Geometry: final body of the model. Coordinates: model frame, mm. A direction names the side the tool comes from. Coordinates: 2 decimals unless noted, no trailing zeros. Order: outer loops, then holes, each group sorted by start corner. A loop starts at its lowest first (then second) coordinate and runs counter-clockwise, first axis right, second up. Notation, with made-up numbers: M -40,67 L -9,67 A21 cw -9,81 Z; hole C 5.25,56.25 d7. An arc over 180 degrees is marked long. Write item = value, one per line.
from build123d import *

# Parameters (mm, degrees)
SKETCH1_R           = 17.35
BOSS_EXTRUDE1_DEPTH = 2.5
SKETCH2_R           = 4.35
CUT_EXTRUDE1_DEPTH  = 25.663637201
SKETCH3_R           = 1.25
CUT_EXTRUDE2_DEPTH  = 25.663637201
CUT_EXTRUDE3_DEPTH  = 25.663637201


with BuildPart() as part:
    # Sketch1 → Boss-Extrude1 (new body)
    with BuildSketch(Plane(origin=(0, 0, 0), x_dir=(1, 0, 0), z_dir=(0, 1, 0))):
        with Locations(Location((0, 0, 0), (0, 0, 270))):
            Circle(SKETCH1_R)
    extrude(amount=BOSS_EXTRUDE1_DEPTH)

    # Sketch2 → Cut-Extrude1 (cut, through all)
    with BuildSketch(Plane(origin=(0, 2.5, 0), x_dir=(1, 0, 0), z_dir=(0, 1, 0))):
        with Locations(Location((0, 0, 0), (0, 0, 270))):
            Circle(SKETCH2_R)
    extrude(amount=-CUT_EXTRUDE1_DEPTH, mode=Mode.SUBTRACT)

    # Sketch3 → Cut-Extrude2 (cut, through all)
    with BuildSketch(Plane(origin=(0, 2.5, 0), x_dir=(1, 0, 0), z_dir=(0, 1, 0))):
        with Locations(Location((-14.5, 0, 0), (0, 0, 270))):
            Circle(SKETCH3_R)
        with Locations(Location((14.5, 0, 0), (0, 0, 270))):
            Circle(SKETCH3_R)
    extrude(amount=-CUT_EXTRUDE2_DEPTH, mode=Mode.SUBTRACT)

    # Sketch4 → Cut-Extrude3 (cut, through all)
    with BuildSketch(Plane(origin=(0, 2.5, 0), x_dir=(1, 0, 0), z_dir=(0, 1, 0))):
        with BuildLine():
            Line((-4, -1.7095321), (-10, -14.17824037))
            ThreePointArc((-10, -14.17824037), (0, -17.35), (10, -14.17824037))
            Line((10, -14.17824037), (4, -1.7095321))
            ThreePointArc((4, -1.7095321), (0, -4.35), (-4, -1.7095321))
        make_face()
    extrude(amount=-CUT_EXTRUDE3_DEPTH, mode=Mode.SUBTRACT)


solid = part.part
1) Line query: L1, parallel to X at y = 1.95, z = 0; L2, parallel to X at y = 0.6, z = -0.5; L3, parallel to X at y = 0.7, z = 11. Output: solid intervals per line, ascending.
Numbers:
L1 = -17.35 to -15.75, -13.25 to -4.35, 4.35 to 13.25, 15.75 to 17.35
L2 = -17.34 to -15.65, -13.35 to -4.32, 4.32 to 13.35, 15.65 to 17.34
L3 = -13.42 to -8.47, 8.47 to 13.42
2) Set-up query: faces 1 (the face through (7.04, 1.27, 8.03)), 2 (the face through (15.74, 1.27, -0.16)). Return all of +Z, -Z, +X, -X, +Y, -Y with unobstructed straight access to the full face (end or side cutting, diameter ignored); none if empty.
Numbers:
face_1 = +Z, +Y, -Y
face_2 = +Y, -Y
3) Section B-B, the plane x = 14.5. Return loops of the section in (y, z), and give its area (3 significant figures).
Numbers:
outline = M 0,-9.53 L 2.5,-9.53 L 2.5,-1.25 L 0,-1.25 Z; M 0,1.25 L 2.5,1.25 L 2.5,9.53 L 0,9.53 Z
area = 41.4 mm²
4) Section A-A, the plane z = 0. Return loops of the section in (x, y), and give its area (3 significant figures).
Numbers:
outline = M -17.35,0 L -15.75,0 L -15.75,2.5 L -17.35,2.5 Z; M -13.25,0 L -4.35,0 L -4.35,2.5 L -13.25,2.5 Z; M 4.35,0 L 13.25,0 L 13.25,2.5 L 4.35,2.5 Z; M 15.75,0 L 17.35,0 L 17.35,2.5 L 15.75,2.5 Z
area = 52.5 mm²
5) Mould query, pull axis X, two halves, no side actions, for faces 3 (the face through (-13.26, 1.27, -0.16)), 4 (the face through (0.61, 1.23, -17.34)), 5 (the face through (-6.96, 1.27, 7.86)), 6 (the face through (0, 2.5, -5)). Classes: pulls with the +X half, pulls with the -X half, needs draft (parallel to the pull), parting line crosses it, or undercut.
Numbers:
face_3 = undercut
face_4 = parting line crosses it
face_5 = undercut
face_6 = needs draft
6) Section C-C, the plane z = 8. Return loops of the section in (x, y).
Numbers:
outline = M -15.4,0 L -7.03,0 L -7.03,2.5 L -15.4,2.5 Z; M 7.03,0 L 15.4,0 L 15.4,2.5 L 7.03,2.5 Z
7) Pin query (flat end, axial travel): pin 1 (5 mm diameter, centred on x = 0, z = 0, fed in from -Y); pin 2 (1 mm diameter, centred on y = 1, z = -3.5, fed in from -X). Return the tip coordinate at first contact, or that it passes through.
Numbers:
pin_1 = through
pin_2 = -17.09
8) Section D-D, the plane y = 0.4. Return loops of the section in (x, z).
Numbers:
outline = M -10,14.18 A17.35 ccw long 10,14.18 L 4,1.71 A4.35 cw long -4,1.71 Z; hole C -14.5,0 d2.5; hole C 14.5,0 d2.5
